Model file for the job. Use its own axes, mm. A direction names the side the tool comes from. Give positions to 0.01 mm unless a question says otherwise; leave off trailing zeros. Order: outer loops, then holes, each group sorted by start corner. A loop starts at its lowest first (then second) coordinate and runs counter-clockwise, first axis right, second up. Notation, with made-up numbers: M 15.5,75 L 60.5,75 A10 ccw 60.5,85 Z; hole C -15,52 d2. An arc over 180 degrees is marked long. Return JSON: item names as keys, results as strings. Group by question number.
1. Slice it at B-B on z = 0. List the corners of the cut face in (x, y).
2. Slice it at A-A on x = 32. List the corners of the cut face in (y, z).
3. Wall check: probe 1 along X at (y, z) = (11.15, 0); probe 2 along X at (y, z) = (8, 16); probe 3 along X at (y, z) = (9.75, 30.5). Give the ranges that are in metal, low to high. Write a range as [from, to].
4. Two-plate mould, pull along X, no slides. Class faces 3 (the face through (1, 0, -2)), 4 (the face through (7.629, 10.196, 72.065)), 5 (the face through (-46.125, 6.261, -61.007)): released by +X, released by -X, zero draft, split by the parting line, or undercut.
5. 3-axis set-ups, long thin cutter, end or side, ignore diameter. For faces 1 (the face through (1, 12.7, -2)), 2 (the face through (48, 7.62, 0)): which of +Z, -Z, +X, -X, +Y, -Y reach the whole face in a straight line?
6. Slice it at C-C on y = 2.25. List the corners of the cut face in (x, z), then the cut area to 3 significant figures.
7. Pin check, flat tips, straight feed: pin 1 (15 mm diameter, centred on x = -12, z = -48, fed in from +Y); pin 2 (6 mm diameter, centred on y = 9, z = 23, fed in from +X); pin 3 (2 mm diameter, centred on x = -22.5, y = 2.5, fed in from -Z). Stop position of each tip, or through.
8. Slice it at D-D on z = -34.5. List the corners of the cut face in (x, y), then the cut area to 3 significant figures.
from build123d import *

# Parameters (mm, degrees)
SKETCH1_R           = 76.227284409
BOSS_EXTRUDE1_DEPTH = 12.7
SKETCH5_R           = 25.4
CUT_EXTRUDE2_DEPTH  = 5.08
SKETCH7_R           = 25.4
CUT_EXTRUDE4_DEPTH  = 5.08


with BuildPart() as part:
    # Sketch1 → Boss-Extrude1 (new body)
    with BuildSketch(Plane(origin=(0, 0, 0), x_dir=(1, 0, 0), z_dir=(0, 1, 0))):
        with Locations(Location((0.257754177, 0.515508354, 0), (0, 0, 270))):
            Circle(SKETCH1_R)
    extrude(amount=BOSS_EXTRUDE1_DEPTH)

    # Sketch5 → Cut-Extrude2 (cut)
    with BuildSketch(Plane(origin=(0, 12.7, 0), x_dir=(1, 0, 0), z_dir=(0, 1, 0))):
        with Locations(Location((-47.837919056, 0, 0), (0, 0, 270))):
            Circle(SKETCH5_R)
    extrude(amount=-CUT_EXTRUDE2_DEPTH, mode=Mode.SUBTRACT)

    # Sketch7 → Cut-Extrude4 (cut)
    with BuildSketch(Plane(origin=(0, 12.7, 0), x_dir=(1, 0, 0), z_dir=(0, 1, 0))):
        with Locations(Location((0, 47.837919056, 0), (0, 0, 270))):
            Circle(SKETCH7_R)
        with Locations(Location((47.837919056, 0, 0), (0, 0, 270))):
            Circle(SKETCH7_R)
        with Locations(Location((0, -47.837919056, 0), (0, 0, 270))):
            Circle(SKETCH7_R)
    extrude(amount=-CUT_EXTRUDE4_DEPTH, mode=Mode.SUBTRACT)


solid = part.part
Result:
{
 "1": {"outline": "M -75.97,0 L 76.48,0 L 76.48,12.7 L 73.24,12.7 L 73.24,7.62 L 22.44,7.62 L 22.44,12.7 L -22.44,12.7 L -22.44,7.62 L -73.24,7.62 L -73.24,12.7 L -75.97,12.7 Z"},
 "2": {"outline": "M 0,-69.82 L 12.7,-69.82 L 12.7,-19.86 L 7.62,-19.86 L 7.62,19.86 L 12.7,19.86 L 12.7,68.79 L 0,68.79 Z"},
 "3": {"probe 1": "x = [-75.97, -73.24], [-22.44, 22.44], [73.24, 76.48]", "probe 2": "x = [-74.16, -67.57], [-28.11, 28.11], [67.57, 74.67]", "probe 3": "x = [-69.37, -18.56], [18.56, 69.89]"},
 "4": {"face 3": "zero draft", "face 4": "undercut", "face 5": "split by the parting line"},
 "5": {"face 1": "+Z, -Z, +X, -X, +Y", "face 2": "+Y"},
 "6": {"outline": "C 0.26,-0.52 d152.45", "area": "18,300 mm2"},
 "7": {"pin 1": "stops at y = 7.62", "pin 2": "stops at x = 73.67", "pin 3": "stops at z = -73.57"},
 "8": {"outline": "M -67.97,0 L 68.49,0 L 68.49,12.7 L 21.62,12.7 L 21.62,7.62 L -21.62,7.62 L -21.62,12.7 L -67.97,12.7 Z", "area": "1,510 mm2"}
}
